Could you check a few things on this model? Use its own coordinates, in mm. A direction names the side the tool comes from. Give positions to 0.01 mm unless a question says otherwise; leave off trailing zeros. Order: outer loops, then holes, each group sorted by start corner. A loop starts at its lowest first (then second) coordinate and runs counter-clockwise, first axis right, second up.
(1) Imagine slicing it at A-A, the plane x = 0. State how many separate pieces and enclosed holes the cut face has, then the cut area to 3 significant figures.
(2) Will these pins go through, and if not, where does the flat tip stop? pin 1 (4 mm diameter, centred on x = 7.5, y = -9, fed in from -Z); pin 2 (2 mm diameter, centred on x = -3, z = -2.5, fed in from -Y); pin 3 (1.2 mm diameter, centred on x = 0, z = -1, fed in from -Y); pin 4 (4 mm diameter, centred on x = -8.5, y = -9, fed in from -Z).
(3) If I drill on probe 1 along X at (y, z) = (2.75, 11.75); probe 2 along Y at (x, z) = (5, 10.25); probe 3 along X at (y, z) = (5, 9.25), over which ranges is the centre line in solid material (lowest first)?
(4) Imagine slicing it at B-B, the plane z = 10.5. Write out the boundary of the cut face in (x, y).
(5) On a 3-axis mill with a long thin cutter (end or side, diameter ignored), from which of +Z, -Z, +X, -X, +Y, -Y can I reach the whole of each face in a straight line? I mean faces 1 (the flat face through (0, 12.349, 7)), 2 (the flat face through (0, 0, 5.08)), 3 (the flat face through (6.436, 0, 9)), 4 (the cylindrical face through (7.276, 9.217, -1.252)), 5 (the cylindrical face through (0.06, -0.08, -2.61)). Say none if no direction works.
(6) If we mould it in two halves opening along Y, with no side actions, what happens to faces 6 (the cylindrical face through (0.157, -11.967, 0.362)), 7 (the cylindrical face through (0.134, -0.458, -6.086)), 8 (the cylindrical face through (-8.862, 6.767, 1.252))? For each: released by +Y, released by -Y, zero draft, split by the parting line, or undercut.
(7) Imagine slicing it at C-C, the plane x = 5. Write out the boundary of the cut face in (y, z), then the cut area to 3 significant figures.
(8) Imagine slicing it at D-D, the plane z = -5. Write out the boundary of the cut face in (x, y), then the cut area to 3 significant figures.
from build123d import *

# Parameters (mm, degrees)
F0_W      = 24.9930880964
F0_H      = 24.6987380087
F1_DEPTH  = 12.7
F2_W      = 19.1328264773
F2_H      = 18.4370856732
F3_DEPTH  = 2.54
F4_W      = 12.8711769357
F4_H      = 12.8711741418
F5_DEPTH  = 2.54
F6_W      = 6.6095204093
F6_H      = 6.6095213406
F7_DEPTH  = 2.54
F8_W      = 1.3914771844
F8_H      = 13.9147825539
F9_ANGLE  = 180
F10_W     = 1.0436060838
F10_H     = 9.0446090326
F12_W     = 2.4350825697
F12_H     = 2.9568914324
F13_ANGLE = 180
F14_R     = 1.27
F15_R     = 1.27
F16_R     = 1.27
F17_R     = 1.27
F18_R     = 1.7737932194
F18_R_2   = 1.7435308636
F19_DEPTH = 2.54
F18_R_3   = 1.7420613373
F18_R_4   = 1.7737943152
F20_DEPTH = 2.54
F22_DEPTH = 2.54
F24_DEPTH = 2.54


with BuildPart() as f1:
    # F0 (on Top) → F1 (new body)
    with BuildSketch(Plane.XY):
        Rectangle(F0_W, F0_H)
    extrude(amount=F1_DEPTH)

    # F2 (on face) → F3 (cut)
    with BuildSketch(Plane.XY.offset(12.7)):
        Rectangle(F2_W, F2_H)
    extrude(amount=-F3_DEPTH, mode=Mode.SUBTRACT)

    # F4 (on face) → F5 (cut)
    with BuildSketch(Plane.XY.offset(10.16)):
        Rectangle(F4_W, F4_H)
    extrude(amount=-F5_DEPTH, mode=Mode.SUBTRACT)

    # F6 (on face) → F7 (cut)
    with BuildSketch(Plane.XY.offset(7.62)):
        Rectangle(F6_W, F6_H)
    extrude(amount=-F7_DEPTH, mode=Mode.SUBTRACT)

    # F8 (on Top) → F9 (revolve)
    with BuildSketch(Plane.XY):
        with Locations((3.304760321, -0.1739347354)):
            Rectangle(F8_W, F8_H)
    revolve(axis=Axis((0, -0.1739347354, 0), (0, 1, 0)), revolution_arc=F9_ANGLE)

    # F10 (on Top) → F11 (revolve)
    with BuildSketch(Plane.XY):
        with Locations((6.6095206421, -0.5218042061)):
            Rectangle(F10_W, F10_H)
    revolve(axis=Axis((0, -0.8696736768, 0), (0, 1, 0)))

    # F12 (on Top) → F13 (revolve)
    with BuildSketch(Plane.XY):
        with Locations((9.392477572, -1.4784457162)):
            Rectangle(F12_W, F12_H)
    revolve(axis=Axis((0, -0.5218046717, 0), (0, 1, 0)), revolution_arc=F13_ANGLE)

    # F14
    f14_edges = [f1.edges().sort_by_distance(p)[0] for p in [
        (0, -12.349369, 0),
    ]]
    fillet(f14_edges, radius=F14_R)

    # F15
    f15_edges = [f1.edges().sort_by_distance(p)[0] for p in [
        (-12.496544, 0.635, 0),
    ]]
    fillet(f15_edges, radius=F15_R)

    # F16
    f16_edges = [f1.edges().sort_by_distance(p)[0] for p in [
        (0.635, 12.349369, 0),
    ]]
    fillet(f16_edges, radius=F16_R)

    # F17
    f17_edges = [f1.edges().sort_by_distance(p)[0] for p in [
        (12.496544, 0, 0),
    ]]
    fillet(f17_edges, radius=F17_R)

    # F18 (on Top) → F19 (join)
    with BuildSketch(Plane.XY):
        with Locations((-8.5228066891, -8.5228048265)):
            Circle(F18_R)
        with Locations((7.5027854182, 7.4880854227)):
            Circle(F18_R_2)
    extrude(amount=-F19_DEPTH)

    # F18 (on Top) → F20 (cut)
    with BuildSketch(Plane.XY):
        with Locations((-7.4791945517, 7.8270649537)):
            Circle(F18_R_3)
        with Locations((7.8270649537, -8.5228048265)):
            Circle(F18_R_4)
    extrude(amount=F20_DEPTH, mode=Mode.SUBTRACT)

    # F21 (on face) → F22 (cut)
    with BuildSketch(Plane.YZ.offset(12.4965440482)):
        with BuildLine():
            add(Edge.make_bspline(
                [(7.4816909619, 6.3803573139), (8.6678256626, 7.222641581), (0.0654100682, 10.7050572044), (-15.1471126917, 6.1563977773), (5.8379660659, 5.2131343851), (7.4816909619, 6.3803573139)],
                knots=[0, 0, 0, 0, 0.294675987, 0.5916431282, 1, 1, 1, 1], degree=3))
        make_face()
    extrude(amount=-F22_DEPTH, mode=Mode.SUBTRACT)

    # F23 (on face) → F24 (cut)
    with BuildSketch(Plane(origin=(-12.4965440482, 0, 0), x_dir=(0, -1, 0), z_dir=(-1, 0, 0))):
        with BuildLine():
            add(Edge.make_bspline(
                [(-7.4785943143, 6.1592552811), (-8.7327498412, 7.2143790552), (-0.1044548846, 11.5753450744), (15.146698404, 5.8495465933), (-5.7683471063, 4.7204205831), (-7.4785943143, 6.1592552811)],
                knots=[0, 0, 0, 0, 0.2971718348, 0.5947573567, 1, 1, 1, 1], degree=3))
        make_face()
    extrude(amount=-F24_DEPTH, mode=Mode.SUBTRACT)


solid = f1.part
Answer block:
1. separate pieces: 4
1. enclosed holes: 1
1. area: 260 mm2
2. pin 1: stops at z = 0
2. pin 2: stops at y = -7.13
2. pin 3: passes through
2. pin 4: stops at z = -2.54
3. probe 1: x = -12.5 to -9.57, 9.57 to 12.5
3. probe 2: y = -12.35 to -9.22, 9.22 to 12.35
3. probe 3: x = -12.5 to -6.44, 6.44 to 12.5
4. outline: (-12.5, -11.08) arc R1.27 ccw to (-11.23, -12.35) - (11.23, -12.35) arc R1.27 ccw to (12.5, -11.08) - (12.5, 11.08) arc R1.27 ccw to (11.23, 12.35) - (-11.23, 12.35) arc R1.27 ccw to (-12.5, 11.08) - close; hole (-9.57, -9.22) - (9.57, -9.22) - (9.57, 9.22) - (-9.57, 9.22) - close
5. face 1: +Z, -Z, +X, -X, +Y
5. face 2: none
5. face 3: +Z
5. face 4: -Z
5. face 5: +Y, -Y
6. face 6: released by -Y
6. face 7: zero draft
6. face 8: undercut
7. outline: (-12.35, 1.27) arc R1.27 ccw to (-11.08, 0) - (11.08, 0) arc R1.27 ccw to (12.35, 1.27) - (12.35, 12.7) - (9.22, 12.7) - (9.22, 10.16) - (6.44, 10.16) - (6.44, 7.62) - (-6.44, 7.62) - (-6.44, 10.16) - (-9.22, 10.16) - (-9.22, 12.7) - (-12.35, 12.7) - close; (-5.04, -5.08) - (4, -5.08) - (4, -3.47) - (-5.04, -3.47) - close; (-2.96, -9.36) - (0, -9.36) - (0, -6.47) - (-2.96, -6.47) - close
7. area: 257 mm2
8. outline: (-9.36, -2.96) - (-6.47, -2.96) - (-6.47, 0) - (-9.36, 0) - close; (-5.08, -5.04) - (-3.47, -5.04) - (-3.47, 4) - (-5.08, 4) - close; (3.47, -5.04) - (5.08, -5.04) - (5.08, 4) - (3.47, 4) - close; (6.47, -2.96) - (9.36, -2.96) - (9.36, 0) - (6.47, 0) - close
8. area: 46.3 mm2
